Can you work these out from the drawing? Everything is in mm from the part's minimum corner. A direction names the side the tool comes from. Give positions to 0.01 mm unless a question says otherwise; leave off trailing zeros. Order: outer loops, then holes, each group sorted by start corner. A loop starts at its lowest first (then second) coordinate and runs counter-clockwise, first axis right, second up. Notation, with made-up numbers: (12, 73.5) - (55, 73.5) arc R19 ccw to (55, 100.5) - close; hole circle Ø3 at (-37.5, 83). An arc over 180 degrees is marked (long way). Answer as a JSON object with one key per item and string values.
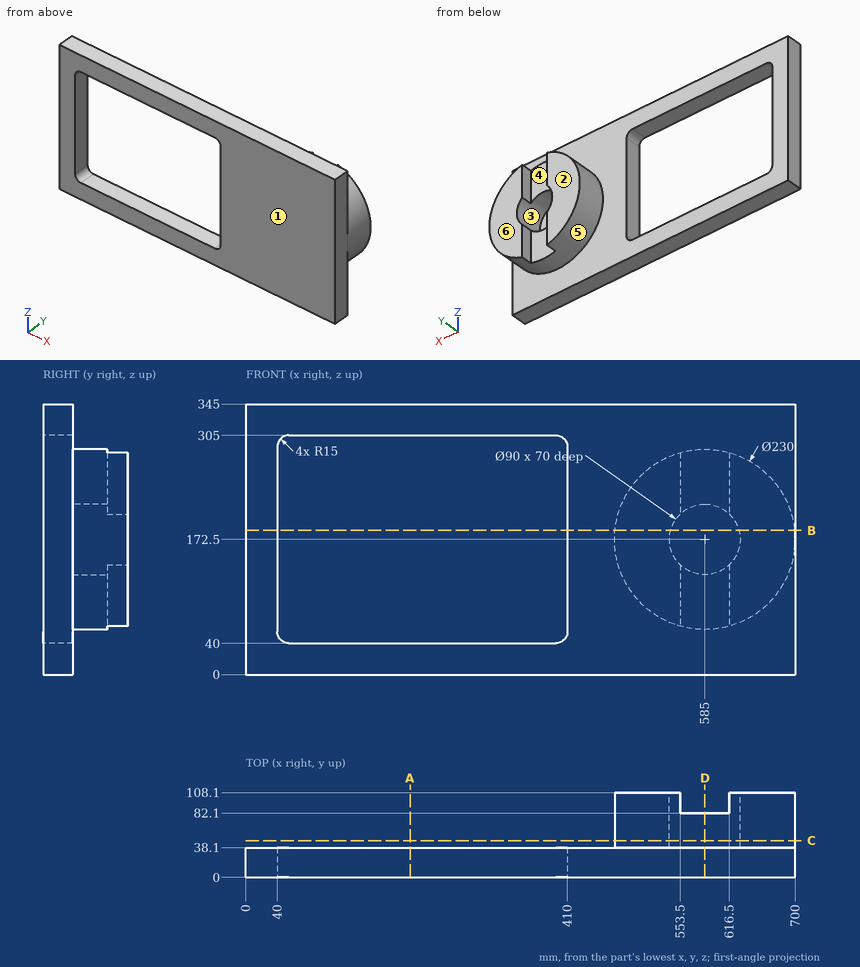
Q1. Which directions (+Z, -Z, +X, -X, +Y, -Y) give clear straight access to the entire face, cutting with the end or side of a thin tool? Please do the marked faces 4, 5 and 6.
Recorded:
{"face 4": "+Z, -Z, +Y", "face 5": "+Y", "face 6": "+Z, -Z, +X, -X, +Y"}
Q2. We'd pull the mould along Y, two halves only. Please class the marked faces 1, 2 and 3: released by +Y, released by -Y, zero draft, split by the parting line, or undercut.
Recorded:
{"face 1": "released by -Y", "face 2": "released by +Y", "face 3": "zero draft"}
Q3. I need wall thicknesses on L1, parallel to X at y = 61, z = 172.5; L2, parallel to X at y = 8, z = 275.5; L3, parallel to Z at x = 585, y = 80. Which ranges of each line are inside material? Lowest first, please.
Recorded:
{"L1": "x = 470 to 540, 630 to 700", "L2": "x = 0 to 40, 410 to 700", "L3": "z = 57.5 to 127.5, 217.5 to 287.5"}
Q4. If we section it at D-D, the plane x = 585: Please give me the cut outline in (y, z).
Recorded:
{"outline": "(0, 0) - (38.1, 0) - (38.1, 57.5) - (82.1, 57.5) - (82.1, 127.5) - (38.1, 127.5) - (38.1, 217.5) - (82.1, 217.5) - (82.1, 287.5) - (38.1, 287.5) - (38.1, 345) - (0, 345) - close"}
Q5. If we section it at C-C, the plane y = 47: Please give me the cut outline in (x, z), then the cut area to 3 significant figures.
Recorded:
{"outline": "circle Ø230 at (585, 172.5); hole circle Ø90 at (585, 172.5)", "area": "35,200 mm^2"}
Q6. If we section it at A-A, the plane x = 209.5: Please give me the cut outline in (y, z), then the cut area to 3 significant figures.
Recorded:
{"outline": "(0, 0) - (38.1, 0) - (38.1, 40) - (0, 40) - close; (0, 305) - (38.1, 305) - (38.1, 345) - (0, 345) - close", "area": "3,050 mm^2"}
Q7. I'm going to push flat-ended pins straight in: pin 1 Ø13 at (y, z) = (89.5, 112) entering from -X; pin 2 Ø21 at (y, z) = (99.5, 236) entering from -X; pin 3 Ø21 at (y, z) = (97.5, 82.5) entering from +X. Where does each tip first touch, or does it pass through?
Recorded:
{"pin 1": "stops at x = 483.47", "pin 2": "stops at x = 482.94", "pin 3": "stops at x = 668.09"}
Q8. If we section it at B-B, the plane z = 184: Please give me the cut outline in (x, y).
Recorded:
{"outline": "(0, 0) - (40, 0) - (40, 38.1) - (0, 38.1) - close; (410, 0) - (700, 0) - (700, 38.1) - (699.42, 38.1) - (699.42, 108.1) - (628.51, 108.1) - (628.51, 38.1) - (541.49, 38.1) - (541.49, 108.1) - (470.58, 108.1) - (470.58, 38.1) - (410, 38.1) - close"}
